Verification items for the finished model (mm, model axes). Give positions to 0.01 mm unless a question says otherwise; leave off trailing zeros. Order: outer loops, then holes, each group sorted by start corner. A loop starts at its lowest first (then second) coordinate and runs counter-clockwise, first axis right, second up. Notation, with made-up numbers: (-29.5, 25) -> (10.5, 25) arc R37 ccw to (10.5, 63) -> close; hole circle Ø4 at (23, -10). An arc over 180 degrees is marked (long way). Write each question's results on one line, items separated by ' | '. Start each with the question number.
1. Cross-section at B-B, the plane y = 17.5. Enter the section's corners in (x, z).
2. Depth check by flat-ended pin: pin 1 Ø3.5 at (y, z) = (91, 2.5) entering from +X; pin 2 Ø12 at (x, y) = (139, 16) entering from +Z; pin 3 Ø3 at (x, z) = (133, 4.5) entering from -Y; pin 4 Ø3 at (x, z) = (134, 3.5) entering from +Y. Enter the tip coordinate at first touch or a pass-through.
3. Cross-section at A-A, the plane x = 141. Enter the section's corners in (y, z).
4. Cross-section at D-D, the plane y = 77. Enter the section's corners in (x, z).
5. Material ranges on L1, parallel to Y at x = 80, z = 5.15; L2, parallel to X at y = 20.5, z = 1; L3, parallel to Y at x = 187, z = 1.4, recorded low to high. Write a range as from..to.
from build123d import *

# Parameters (mm, degrees)
SKETCH_1_W      = 204
SKETCH_1_H      = 30
EXTRUDE_1_DEPTH = 6
FILLET_1_R      = 6


with BuildPart() as part:
    # Эскиз1 → Бобышка-Вытянуть1 (new body)
    with BuildSketch(Plane.XY):
        Polygon((0, 20), (0, 0), (97, 0), (97, 6), (147, 6), (147, 0), (244, 0), (244, 20), (250, 20), (250, 40), (244, 40), (244, 90), (220, 90), (220, 93), (161, 93), (161, 87), (164, 87), (164, 60), (154, 60), (154, 54), (124, 54), (124, 60), (0, 60), (0, 40), (-6, 40), (-6, 20), align=None)
        with Locations((122, 30)):
            Rectangle(SKETCH_1_W, SKETCH_1_H, mode=Mode.SUBTRACT)
    extrude(amount=EXTRUDE_1_DEPTH)

    # Скругление1
    fillet_1_edges = [part.edges().sort_by_distance(p)[0] for p in [
        (161, 93, 3),
    ]]
    fillet(fillet_1_edges, radius=FILLET_1_R - 0.0001)  # a hair under: the kernel refuses the full size


solid = part.part
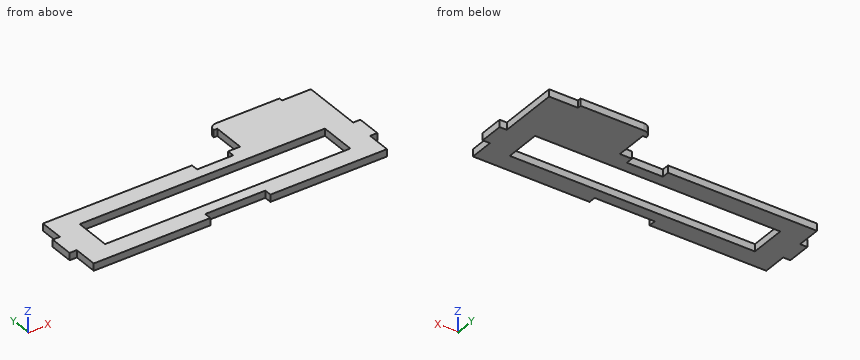
Results below:
1) outline: (0, 0) -> (20, 0) -> (20, 6) -> (0, 6) -> close; (224, 0) -> (244, 0) -> (244, 6) -> (224, 6) -> close
2) pin 1: stops at x = 244 | pin 2: stops at z = 6 | pin 3: stops at y = 6 | pin 4: stops at y = 54
3) outline: (6, 0) -> (15, 0) -> (15, 6) -> (6, 6) -> close; (45, 0) -> (54, 0) -> (54, 6) -> (45, 6) -> close
4) outline: (164, 0) -> (244, 0) -> (244, 6) -> (164, 6) -> close
5) L1: y = 0..15, 45..60 | L2: x = -6..20, 224..250 | L3: y = 0..15, 45..93
